Check sheet for the modelled part. Datum: model origin and axes. Units: mm. A direction names the side the tool comes from. Give positions to 0.01 mm unless a question says otherwise; leave off trailing zeros. Write each loop counter-clockwise with the first axis right and the second up, starting at its lowest first coordinate (ties: lowest second). Pieces come first, ordered by that corner, then holes. Notation, with made-up numbers: M 17.5,37 L 28.5,37 A13 cw 28.5,51 Z; hole C 1.5,81 d2. An arc over 180 degrees is marked long. Write item = value, one per line. Start each with the question number.
1) Access from +Z, -Z, +X, -X, +Y, -Y to the whole of each face (thin tool, end or side, straight path). Record for faces 4 (the flat face through (-32.105, 2, -29)), 5 (the flat face through (-30, 4.56, -12)), 6 (the flat face through (-30, 4.56, -29)), 7 (the flat face through (-27.295, 2, -29)).
2) Cross-section at D-D, the plane y = 3.2. Give the number of separate pieces and of enclosed holes in the cut face, plus the area to 3 significant figures.
3) Scan lines: line 1 along Z through (x, y) = (-16, 1.15) (1 decimal); line 2 along Z through (x, y) = (-39, 2.25) (1 decimal); line 3 along X through (y, z) = (1.1, -19.5). Record each from-to range of solid material in increasing order. Write a range as [from, to].
4) Cross-section at A-A, the plane z = 0. Record the cut outline in (x, y) (1 decimal), plus the area to 3 significant figures.
5) Mould release check, pull along X, two halves, no side actions. Record for faces 1 (the flat face through (40, 2, -45.238)), 2 (the flat face through (50, 2, 40)), 3 (the flat face through (-7, 2, -23.207)): released by +X, released by -X, zero draft, split by the parting line, or undercut.
6) Cross-section at C-C, the plane x = 0. Record the cut outline in (y, z) (1 decimal), plus the area to 3 significant figures.
7) Cross-section at B-B, the plane x = -41.5. Record the cut outline in (y, z) (1 decimal).
8) Go/stop test with flat-tipped pins: pin 1 (4 mm diameter, centred on x = -29, z = -12, fed in from +Y); pin 2 (2.5 mm diameter, centred on y = 1, z = 48.5, fed in from -X); pin 3 (8 mm diameter, centred on x = -37.5, z = 4.5, fed in from -Y); pin 4 (2.5 mm diameter, centred on x = -48.5, y = 2.5, fed in from +Z). Record where each tip stops, or that it passes through.
```python
from build123d import *

# Parameters (mm, degrees)
SKETCH1_W           = 100
SKETCH1_H           = 100
BOSS_EXTRUDE1_DEPTH = 4.7625
SKETCH2_W           = 20
SKETCH2_H           = 4.7625
SKETCH2_W_2         = 4.7625
SKETCH2_H_2         = 20
CUT_EXTRUDE1_DEPTH  = 4.7625
SKETCH3_R           = 9.525
CUT_EXTRUDE2_DEPTH  = 71.870878407
CAVITY2_START       = -14.7625
CAVITY2_DEPTH       = 4.810125
CAVITY2_START_2     = -31.725
CAVITY2_2_DEPTH     = 4.810125
CAVITY2_START_3     = -23.2065625
CAVITY2_3_OUTLINE_W = 4.810125
CAVITY2_3_OUTLINE_H = 4.7625
CAVITY2_3_DEPTH     = 4.810125
CAVITY2_START_4     = -26.914875
CAVITY2_4_OUTLINE_W = 4.810125
CAVITY2_4_OUTLINE_H = 0.203
CAVITY2_4_DEPTH     = 12.152375


# Read off the part's stored shape, not the designer's step: Cavity2
with BuildPart() as part:
    # Sketch1 → Boss-Extrude1 (new body)
    with BuildSketch(Plane(origin=(0, 0, 0), x_dir=(1, 0, 0), z_dir=(0, 1, 0))):
        Rectangle(SKETCH1_W, SKETCH1_H)
    extrude(amount=BOSS_EXTRUDE1_DEPTH)

    # Sketch2 → Cut-Extrude1 (cut)
    with BuildSketch(Plane(origin=(0, 4.7625, 0), x_dir=(1, 0, 0), z_dir=(0, 1, 0))):
        Polygon((-50, 45.2375), (-45.2375, 45.2375), (-30, 45.2375), (-30, 50), (-50, 50), align=None)
        with Locations((0, 47.61875)):
            Rectangle(SKETCH2_W, SKETCH2_H)
        Polygon((30, 50), (30, 45.2375), (45.2375, 45.2375), (50, 45.2375), (50, 50), align=None)
        with Locations((47.61875, 15.2375)):
            Rectangle(SKETCH2_W_2, SKETCH2_H_2)
        with Locations((47.61875, -24.7625)):
            Rectangle(SKETCH2_W_2, SKETCH2_H_2)
        Polygon((45.2375, -45.2375), (30, -45.2375), (30, -50), (50, -50), (50, -45.2375), align=None)
        with Locations((0, -47.61875)):
            Rectangle(SKETCH2_W, SKETCH2_H)
        Polygon((-30, -45.2375), (-45.2375, -45.2375), (-50, -45.2375), (-50, -50), (-30, -50), align=None)
        with Locations((-47.61875, -15.2375)):
            Rectangle(SKETCH2_W_2, SKETCH2_H_2)
        with Locations((-47.61875, 24.7625)):
            Rectangle(SKETCH2_W_2, SKETCH2_H_2)
    extrude(amount=-CUT_EXTRUDE1_DEPTH, mode=Mode.SUBTRACT)

    # Sketch3 → Cut-Extrude2 (cut, through all)
    with BuildSketch(Plane(origin=(0, 4.7625, 0), x_dir=(1, 0, 0), z_dir=(0, 1, 0))):
        with Locations(Location((0, 0, 0), (0, 0, 270))):
            Circle(SKETCH3_R)
    extrude(amount=-CUT_EXTRUDE2_DEPTH, mode=Mode.SUBTRACT)

    # Cavity2 outline → Cavity2 (cut)
    with BuildSketch(Plane.XY.offset(CAVITY2_START)):
        Polygon((-4.386875, 4.5595), (-4.386875, 4.7625), (-45.392875, 4.7625), (-45.392875, 0), (-32.1050625, 0), (-32.1050625, 4.5595), (-27.2949375, 4.5595), (-27.2949375, 0), (-14.007125, 0), (-14.007125, 4.5595), align=None)
    extrude(amount=CAVITY2_DEPTH, mode=Mode.SUBTRACT)

    # Cavity2 2 outline → Cavity2 2 (cut)
    with BuildSketch(Plane.XY.offset(CAVITY2_START_2)):
        Polygon((-4.386875, 4.5595), (-4.386875, 4.7625), (-45.2375, 4.7625), (-45.2375, 0), (-32.1050625, 0), (-32.1050625, 4.5595), (-27.2949375, 4.5595), (-27.2949375, 0), (-14.007125, 0), (-14.007125, 4.5595), align=None)
    extrude(amount=CAVITY2_2_DEPTH, mode=Mode.SUBTRACT)

    # Cavity2 3 outline → Cavity2 3 (cut)
    with BuildSketch(Plane.XY.offset(CAVITY2_START_3)):
        with Locations((-6.9949375, 2.38125)):
            Rectangle(CAVITY2_3_OUTLINE_W, CAVITY2_3_OUTLINE_H)
    extrude(amount=CAVITY2_3_DEPTH, mode=Mode.SUBTRACT)

    # Cavity2 4 outline → Cavity2 4 (cut)
    with BuildSketch(Plane.XY.offset(CAVITY2_START_4)):
        with Locations((-6.9949375, 4.661)):
            Rectangle(CAVITY2_4_OUTLINE_W, CAVITY2_4_OUTLINE_H)
    extrude(amount=CAVITY2_4_DEPTH, mode=Mode.SUBTRACT)


solid = part.part
```
Reply:
q1.face_4 = -X, +Y, -Y
q1.face_5 = +Y
q1.face_6 = -X, +Y
q1.face_7 = +Y, -Y
q2.separate_pieces = 1
q2.enclosed_holes = 4
q2.area = 8,480 mm2
q3.line_1 = [-50, -31.7], [-26.9, -14.8], [-10, 50]
q3.line_2 = [-45.2, -31.7], [-26.9, -14.8], [-10, 45.2]
q3.line_3 = [-45.24, -9.4], [-4.59, 45.24]
q4.outline = M -50,0 L -9.5,0 L -9.5,4.8 L -50,4.8 Z; M 9.5,0 L 50,0 L 50,4.8 L 9.5,4.8 Z
q4.area = 386 mm2
q5.face_1 = zero draft
q5.face_2 = released by +X
q5.face_3 = undercut
q6.outline = M 0,-45.2 L 4.8,-45.2 L 4.8,-9.5 L 0,-9.5 Z; M 0,9.5 L 4.8,9.5 L 4.8,45.2 L 0,45.2 Z
q6.area = 340 mm2
q7.outline = M 0,-45.2 L 4.8,-45.2 L 4.8,-31.7 L 0,-31.7 Z; M 0,-26.9 L 4.8,-26.9 L 4.8,-14.8 L 0,-14.8 Z; M 0,-10 L 4.8,-10 L 4.8,45.2 L 0,45.2 Z
q8.pin_1 = 4.56
q8.pin_2 = -30
q8.pin_3 = 0
q8.pin_4 = 45.24
